```python
from build123d import *

# Parameters (mm, degrees)
SKETCH1_W                               = 12.94
SKETCH1_H                               = 7.5
BOSS_EXTRUDE1_DEPTH                     = 5.35
FILLET1_R                               = 0.5
SKETCH2_W                               = 10.34
SKETCH2_H                               = 4.9
CUT_EXTRUDE1_DEPTH                      = 4.35
SKETCH3_W                               = 10.34
SKETCH3_H                               = 1.6
CUT_EXTRUDE2_DEPTH                      = 2
SKETCH4_OUTSIDE_W                       = 18.116
SKETCH4_OUTSIDE_H                       = 10.526
CUT_EXTRUDE3_DEPTH                      = 1.6
FILLET2_R                               = 0.5
CUT_EXTRUDE4_CLEARANCE_FOR_TOP_DEPTH    = 0.05
CUT_EXTRUDE5_CLEARANCE_FOR_BOTTOM_DEPTH = 0.05
CUT_EXTRUDE6_CLEARANCE_ON_SIDES_DEPTH   = 1.7


with BuildPart() as part:
    # Sketch1 → Boss-Extrude1 (new body)
    with BuildSketch(Plane.XY):
        with Locations((0, -0.8)):
            Rectangle(SKETCH1_W, SKETCH1_H)
    extrude(amount=-BOSS_EXTRUDE1_DEPTH)

    # Fillet1
    fillet1_edges = [part.edges().sort_by_distance(p)[0] for p in [
        (-6.47, 2.95, -2.675),
        (6.47, 2.95, -2.675),
        (6.47, -4.55, -2.675),
        (-6.47, -4.55, -2.675),
    ]]
    fillet(fillet1_edges, radius=FILLET1_R)

    # Sketch2 → Cut-Extrude1 (cut)
    with BuildSketch(Plane.XY):
        with Locations((0, -0.8)):
            Rectangle(SKETCH2_W, SKETCH2_H)
    extrude(amount=-CUT_EXTRUDE1_DEPTH, mode=Mode.SUBTRACT)

    # Sketch3 → Cut-Extrude2 (cut, through all)
    with BuildSketch(Plane.XY.offset(-4.35)):
        with Locations((0, -0.8)):
            Rectangle(SKETCH3_W, SKETCH3_H)
    extrude(amount=-CUT_EXTRUDE2_DEPTH, mode=Mode.SUBTRACT)

    # Sketch4 outside → Cut-Extrude3 (cut)
    with BuildSketch(Plane.XZ.offset(1.6)):
        with Locations((0, -2.675)):
            Rectangle(SKETCH4_OUTSIDE_W, SKETCH4_OUTSIDE_H)
        with BuildLine():
            Line((5.97, -3.35), (5.97, 0))
            Line((5.97, 0), (-5.97, 0))
            Line((-5.97, 0), (-5.97, -3.35))
            ThreePointArc((-5.97, -3.35), (-5.677106781, -4.057106781), (-4.97, -4.35))
            Line((-4.97, -4.35), (-4.27, -4.35))
            Line((-4.27, -4.35), (4.27, -4.35))
            Line((4.27, -4.35), (4.97, -4.35))
            ThreePointArc((4.97, -4.35), (5.677106781, -4.057106781), (5.97, -3.35))
        make_face(mode=Mode.SUBTRACT)
    extrude(amount=-CUT_EXTRUDE3_DEPTH, mode=Mode.SUBTRACT)

    # Fillet2
    fillet2_edges = [part.edges().sort_by_distance(p)[0] for p in [
        (6.47, -2.825, -5.35),
        (0, 2.95, -5.35),
        (-6.47, 1.225, -5.35),
        (0, -4.55, -5.35),
        (6.323553391, -4.403553391, -5.35),
        (-6.323553391, -4.403553391, -5.35),
        (-6.323553391, 2.803553391, -5.35),
        (6.323553391, 2.803553391, -5.35),
        (6.47, 1.225, -5.35),
        (-6.47, -2.825, -5.35),
    ]]
    fillet(fillet2_edges, radius=FILLET2_R)

    # Sketch5 → Cut-Extrude4 - clearance for top (cut)
    with BuildSketch(Plane.XZ):
        with BuildLine():
            Line((-5.97, -5.35), (5.97, -5.35))
            ThreePointArc((5.97, -5.35), (6.323553391, -5.203553391), (6.47, -4.85))
            Line((6.47, -4.85), (6.47, 0))
            Line((6.47, 0), (5.97, 0))
            Line((5.97, 0), (5.97, -3.35))
            ThreePointArc((5.97, -3.35), (5.744596669, -3.982455532), (5.17, -4.329795897))
            Line((5.17, -4.329795897), (5.17, -4.35))
            Line((5.17, -4.35), (-5.17, -4.35))
            Line((-5.17, -4.35), (-5.17, -4.329795897))
            ThreePointArc((-5.17, -4.329795897), (-5.744596669, -3.982455532), (-5.97, -3.35))
            Line((-5.97, -3.35), (-5.97, 0))
            Line((-5.97, 0), (-6.47, 0))
            Line((-6.47, 0), (-6.47, -4.85))
            ThreePointArc((-6.47, -4.85), (-6.323553391, -5.203553391), (-5.97, -5.35))
        make_face()
    extrude(amount=-CUT_EXTRUDE4_CLEARANCE_FOR_TOP_DEPTH, mode=Mode.SUBTRACT)

    # Sketch6 → Cut-Extrude5 - clearance for bottom (cut)
    with BuildSketch(Plane(origin=(0, -1.6, 0), x_dir=(1, 0, 0), z_dir=(0, 1, 0))):
        with BuildLine():
            Line((5.97, 5.35), (-5.97, 5.35))
            ThreePointArc((-5.97, 5.35), (-6.323553391, 5.203553391), (-6.47, 4.85))
            Line((-6.47, 4.85), (-6.47, 0))
            Line((-6.47, 0), (-5.97, 0))
            Line((-5.97, 0), (-5.97, 3.35))
            ThreePointArc((-5.97, 3.35), (-5.744596669, 3.982455532), (-5.17, 4.329795897))
            Line((-5.17, 4.329795897), (-5.17, 4.35))
            Line((-5.17, 4.35), (5.17, 4.35))
            Line((5.17, 4.35), (5.17, 4.329795897))
            ThreePointArc((5.17, 4.329795897), (5.744596669, 3.982455532), (5.97, 3.35))
            Line((5.97, 3.35), (5.97, 0))
            Line((5.97, 0), (6.47, 0))
            Line((6.47, 0), (6.47, 4.85))
            ThreePointArc((6.47, 4.85), (6.323553391, 5.203553391), (5.97, 5.35))
        make_face()
    extrude(amount=-CUT_EXTRUDE5_CLEARANCE_FOR_BOTTOM_DEPTH, mode=Mode.SUBTRACT)

    # Sketch7 → Cut-Extrude6 - clearance on sides (cut)
    with BuildSketch(Plane.XZ.offset(-0.05)):
        with BuildLine():
            Line((-5.97, -5.4), (5.97, -5.4))
            ThreePointArc((5.97, -5.4), (6.35890873, -5.23890873), (6.52, -4.85))
            Line((6.52, -4.85), (6.52, 0.05))
            Line((6.52, 0.05), (5.92, 0.05))
            Line((5.92, 0.05), (5.92, -3.35))
            ThreePointArc((5.92, -3.35), (5.692841615, -3.9664414), (5.12, -4.288083152))
            Line((5.12, -4.288083152), (5.12, -4.3))
            Line((5.12, -4.3), (-5.12, -4.3))
            Line((-5.12, -4.3), (-5.12, -4.288083152))
            ThreePointArc((-5.12, -4.288083152), (-5.692841615, -3.9664414), (-5.92, -3.35))
            Line((-5.92, -3.35), (-5.92, 0.05))
            Line((-5.92, 0.05), (-6.52, 0.05))
            Line((-6.52, 0.05), (-6.52, -4.85))
            ThreePointArc((-6.52, -4.85), (-6.35890873, -5.23890873), (-5.97, -5.4))
        make_face()
    extrude(amount=CUT_EXTRUDE6_CLEARANCE_ON_SIDES_DEPTH, mode=Mode.SUBTRACT)


solid = part.part
```
Can you work these out from the model? Positions are in its coordinate system, mm. A direction names the side the tool comes from. Coordinates: 2 decimals unless noted, no trailing zeros. Write each loop counter-clockwise with the first axis right and the second up, starting at its lowest first coordinate (ties: lowest second). Pieces come first, ordered by that corner, then holes. Notation, with made-up numbers: M -34,-26.5 L -22,-26.5 A17 ccw -22,-22.5 Z; hole C 61.25,0 d7. An arc over 180 degrees is marked long. Write item = value, one per line. Start each with the question number.
Q1. If we section it at C-C, the plane z = -1.1: Write out the boundary of the cut face in (x, y), then the cut area to 3 significant figures.
Q2. If we section it at D-D, the plane x = 5.75: Write out the boundary of the cut face in (y, z).
Q3. On a 3-axis mill with a long thin cutter (end or side, diameter ignored), from which of +Z, -Z, +X, -X, +Y, -Y can I reach the whole of each face in a straight line? I mean faces 5 (the face through (0, 1.65, -2)), 6 (the face through (5.92, -1, -2)), 7 (the face through (0, 0.05, -5)). Say none if no direction works.
Q4. If we section it at A-A, the plane y = 0.5: Write out the boundary of the cut face in (x, z).
Q5. If we section it at B-B, the plane x = -3.25: Write out the boundary of the cut face in (y, z), then the cut area to 3 significant figures.
Q6. I'm going to push flat-ended pins straight in: pin 1 (0.5 mm diameter, centred on y = -0.5, z = -1.5, fed in from -X); pin 2 (0.8 mm diameter, centred on x = 0, y = -2, fed in from +Z). Where does each tip first touch, or does it pass through?
Q7. Thinking about a two-plate mould opening in X: for faces 1 (the face through (0, -2, -4.35)), 2 (the face through (0, -1.65, -4.5)), 3 (the face through (0, -3.25, -2)), 4 (the face through (5.715, -0.788, -3.94)), which applies, released by +X, released by -X, zero draft, split by the parting line, or undercut?
Q8. If I drill on L1, parallel to Y at x = -2.5, z = -3.1; L2, parallel to X at y = -0.5, z = -0.8; L3, parallel to Y at x = 0.5, z = -4.7, over which ranges is the centre line in solid material (lowest first)? Write a range as [from, to].
Check sheet entries:
q1.outline = M -6.47,-4.05 A0.5 ccw -5.97,-4.55 L 5.97,-4.55 A0.5 ccw 6.47,-4.05 L 6.47,-1.65 L 5.92,-1.65 L 5.92,0.05 L 6.47,0.05 L 6.47,2.45 A0.5 ccw 5.97,2.95 L -5.97,2.95 A0.5 ccw -6.47,2.45 L -6.47,0.05 L -5.92,0.05 L -5.92,-1.65 L -6.47,-1.65 Z; hole M -5.17,-3.25 L 5.17,-3.25 L 5.17,1.65 L -5.17,1.65 Z
q1.area = 44.3 mm²
q2.outline = M -4.55,-4.85 A0.5 ccw -4.05,-5.35 L -1.65,-5.35 L -1.65,-3.89 L 0.05,-3.89 L 0.05,-5.35 L 2.45,-5.35 A0.5 ccw 2.95,-4.85 L 2.95,0 L -4.55,0 Z
q3.face_5 = +Z
q3.face_6 = +Z, -Z, +X
q3.face_7 = -Z
q4.outline = M -6.47,-4.85 A0.5 ccw -5.97,-5.35 L 5.97,-5.35 A0.5 ccw 6.47,-4.85 L 6.47,0 L 5.17,0 L 5.17,-4.35 L -5.17,-4.35 L -5.17,0 L -6.47,0 Z
q5.outline = M -4.55,-4.85 A0.5 ccw -4.05,-5.35 L -1.65,-5.35 L -1.65,-4.35 L -3.25,-4.35 L -3.25,0 L -4.55,0 Z; M 0.05,-5.35 L 2.45,-5.35 A0.5 ccw 2.95,-4.85 L 2.95,0 L 1.65,0 L 1.65,-4.35 L 0.05,-4.35 Z
q5.area = 17.0 mm²
q6.pin_1 = -5.92
q6.pin_2 = -4.35
q7.face_1 = undercut
q7.face_2 = zero draft
q7.face_3 = undercut
q7.face_4 = released by +X
q8.L1 = [-4.55, -3.25], [1.65, 2.95]
q8.L2 = [-5.92, -5.17], [5.17, 5.92]
q8.L3 = [-4.55, -1.65], [0.05, 2.95]
